Check sheet for the drawn part. Datum: minimum x, y, z corner. Units: mm. Coordinates: 2 decimals unless noted, no trailing zeros. Loops run counter-clockwise (first coordinate to the right, second up) from the corner with the lowest first, then second, coordinate; pieces in that order, holes last.
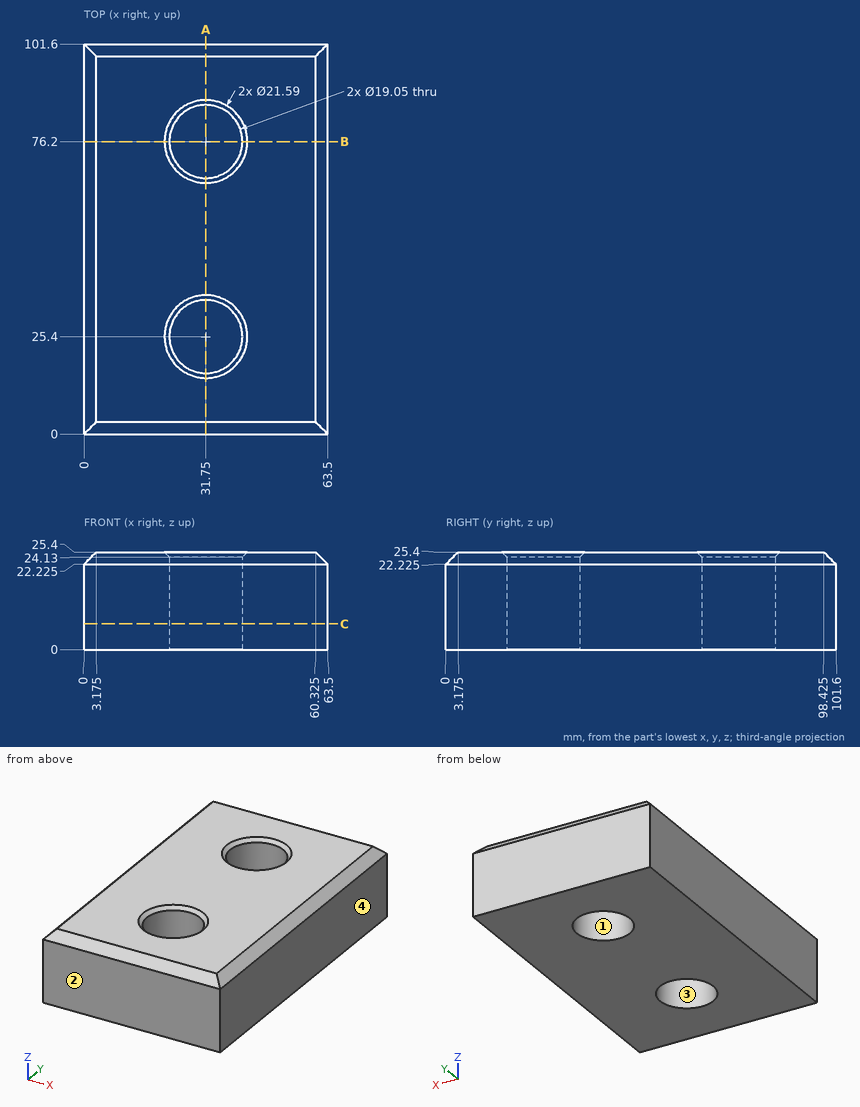
(1) Gauge pin test, flat end, axial feed: pin 1 Ø3 at (y, z) = (35.5, 22.5) entering from +X. Record the tip position at first contact, or that the pin passes through.
Findings:
pin 1: stops at x = 63.5
(2) Sectioned sample at A-A on x = 31.75. Record the cut outline in (y, z) (3 decimals), and give its area (3 significant figures).
Findings:
outline: (0, 0) - (15.875, 0) - (15.875, 24.13) - (14.605, 25.4) - (3.175, 25.4) - (0, 22.225) - close; (34.925, 0) - (66.675, 0) - (66.675, 24.13) - (65.405, 25.4) - (36.195, 25.4) - (34.925, 24.13) - close; (85.725, 0) - (101.6, 0) - (101.6, 22.225) - (98.425, 25.4) - (86.995, 25.4) - (85.725, 24.13) - close
area: 1,600 mm2
(3) Sectioned sample at C-C on z = 6.75. Record the cut outline in (x, y) (3 decimals).
Findings:
outline: (0, 0) - (63.5, 0) - (63.5, 101.6) - (0, 101.6) - close; hole circle Ø19.05 at (31.75, 25.4); hole circle Ø19.05 at (31.75, 76.2)
(4) Scan lines: L1, parallel to Y at x = 31.75, z = 8.25 (3 decimals); L2, parallel to Y at x = 26, z = 20; L3, parallel to X at y = 33, z = 10.25. Record each from-to range of solid material in increasing order.
Findings:
L1: y = 0 to 15.875, 34.925 to 66.675, 85.725 to 101.6
L2: y = 0 to 17.81, 32.99 to 68.61, 83.79 to 101.6
L3: x = 0 to 26.01, 37.49 to 63.5
(5) Sectioned sample at B-B on y = 76.2. Record the cut outline in (x, z) (3 decimals), and give its area (3 significant figures).
Findings:
outline: (0, 0) - (22.225, 0) - (22.225, 24.13) - (20.955, 25.4) - (3.175, 25.4) - (0, 22.225) - close; (41.275, 0) - (63.5, 0) - (63.5, 22.225) - (60.325, 25.4) - (42.545, 25.4) - (41.275, 24.13) - close
area: 1,120 mm2
(6) Draft check along X on the marked faces 1, 2, 3 and 4. Enter one of: +X half, -X half, draft (parallel to the pull), parting line (faces both ways), or undercut.
Findings:
face 1: undercut
face 2: draft
face 3: undercut
face 4: +X half
